Geometry: final body of the model. Coordinates: model frame, mm. A direction names the side the tool comes from. Coordinates: 2 decimals unless noted, no trailing zeros. Loops run counter-clockwise (first coordinate to the right, second up) from the corner with the lowest first, then second, coordinate; pieces in that order, holes last. Notation, with made-up numbers: (10.5, -8) - (31.5, -8) arc R18 cw to (31.5, 8) - close; hole circle Ø11 at (23, 32.5). An arc over 180 degrees is marked (long way). Put each result on its own line as item: value. Start each with the question number.
1) Draft query along Y for faces 5 (the cylindrical face through (0, 3, -22)), 6 (the cylindrical face through (2, 0, -1)), 7 (the flat face through (0, 0, -20)). Return one class per face: +Y half, -Y half, draft (parallel to the pull), parting line (faces both ways), or undercut.
2) Contact query for flat-ended pins moving along their axis: pin 1 Ø3 at (x, y) = (0, 0) entering from +Z; pin 2 Ø3 at (x, z) = (0.5, -19) entering from +Y; pin 3 Ø1.5 at (y, z) = (0.5, -15) entering from +X. Output: stop coordinate, or through.
3) Reachability of faces 1 (the cylindrical face through (0, 2, -28)), 2 (the flat face through (0, 0, -6)), 3 (the cylindrical face through (-3.642, -0.924, 1.117)), 4 (the flat face through (0.1, -2.2, -33)) from +Z, -Z, +X, -X, +Y, -Y: full face, straight path, thin tool, end or side. Return the list, or none.
4) Section B-B on x = 0. Output: boundary loops of the cut face in (y, z).
5) Section A-A on y = 3. Output: boundary loops of the cut face in (x, z), and give its area (3 significant figures).
6) Section C-C on x = -3.5. Output: boundary loops of the cut face in (y, z).
7) Material intervals for line 1 along Z through (x, y) = (0, 3.9); line 2 along Y through (x, z) = (0, -29.75); line 3 along Z through (x, y) = (0.5, -4), sorted ascending. Write a range as from..to.
8) Section D-D on z = -25.5. Output: boundary loops of the cut face in (x, y), and give its area (3 significant figures).
```python
from build123d import *

# Parameters (mm, degrees)
SKETCH1_W                                          = 5.5
SKETCH1_H                                          = 8
SKETCH2_R                                          = 5
BOSS_EXTRUDE1_DEPTH                                = 33
CBORE_FOR_M3_5_HEX_HEAD_MACHINE_SCREW1_D           = 4
CBORE_FOR_M3_5_HEX_HEAD_MACHINE_SCREW1_DEPTH       = 14
CBORE_FOR_M3_5_HEX_HEAD_MACHINE_SCREW1_CBORE_D     = 8.5
CBORE_FOR_M3_5_HEX_HEAD_MACHINE_SCREW1_CBORE_DEPTH = 4
HOLE1_REACH                                        = 38.626
HOLE1_BORE_R                                       = 1
SKETCH6_R                                          = 2
CUT_EXTRUDE1_DEPTH                                 = 10
SKETCH7_R                                          = 2
CUT_EXTRUDE2_DEPTH                                 = 5


with BuildPart() as part:
    # Sketch1 → Revolve1 (revolve)
    with BuildSketch(Plane(origin=(0, 0, 0), x_dir=(1, 0, 0), z_dir=(0, 1, 0))):
        with Locations((2.75, -4)):
            Rectangle(SKETCH1_W, SKETCH1_H)
    revolve(axis=Axis((0, 0, 0), (0, 0, 1)))

    # Sketch2 → Boss-Extrude1 (add)
    with BuildSketch(Plane(origin=(0, 0, 0), x_dir=(-1, 0, 0), z_dir=(0, 0, -1))):
        Circle(SKETCH2_R)
    extrude(amount=BOSS_EXTRUDE1_DEPTH)

    # CBORE for M3.5 Hex Head Machine Screw1
    with Locations(Plane.XY.offset(8)):
        with Locations((0, 0)):
            CounterBoreHole(CBORE_FOR_M3_5_HEX_HEAD_MACHINE_SCREW1_D / 2, CBORE_FOR_M3_5_HEX_HEAD_MACHINE_SCREW1_CBORE_D / 2, CBORE_FOR_M3_5_HEX_HEAD_MACHINE_SCREW1_CBORE_DEPTH, depth=CBORE_FOR_M3_5_HEX_HEAD_MACHINE_SCREW1_DEPTH)

    # Hole1 bore (on position points) → Hole1 (cut, up to next)
    with BuildSketch(Plane(origin=(-5.5, 0, 1.5), x_dir=(0, -1, 0), z_dir=(-1, 0, 0)), mode=Mode.PRIVATE) as hole1_sk1:
        Circle(HOLE1_BORE_R)
    hole1_tool1 = extrude(hole1_sk1.sketch, amount=-HOLE1_REACH, mode=Mode.PRIVATE) & part.part
    add(hole1_tool1.solids().sort_by_distance((-5.5, 0, 1.5))[0], mode=Mode.SUBTRACT)

    # Sketch6 → Cut-Extrude1 (cut)
    with BuildSketch(Plane(origin=(0, 0, -33), x_dir=(-1, 0, 0), z_dir=(0, 0, -1))):
        with Locations(Location((0, 0, 0), (0, 0, 180))):
            Circle(SKETCH6_R)
    extrude(amount=-CUT_EXTRUDE1_DEPTH, mode=Mode.SUBTRACT)

    # Sketch7 → Cut-Extrude2 (cut)
    with BuildSketch(Plane(origin=(0, 5, 0), x_dir=(1, 0, 0), z_dir=(0, 1, 0))):
        with Locations(Location((0, 20, 0), (0, 0, 270))):
            Circle(SKETCH7_R)
    extrude(amount=-CUT_EXTRUDE2_DEPTH, mode=Mode.SUBTRACT)


solid = part.part
```
Answer block:
1. face 5: draft
1. face 6: undercut
1. face 7: +Y half
2. pin 1: stops at z = -6
2. pin 2: stops at y = 5
2. pin 3: stops at x = 5
3. face 1: -Z
3. face 2: +Z
3. face 3: -X
3. face 4: -Z, +X, -X, +Y, -Y
4. outline: (-5.5, 0) - (-5, 0) - (-5, -33) - (-2, -33) - (-2, -23) - (2, -23) - (2, -33) - (5, -33) - (5, -22) - (0, -22) - (0, -18) - (5, -18) - (5, 0) - (5.5, 0) - (5.5, 8) - (4.25, 8) - (4.25, 4) - (2, 4) - (2, -6) - (-2, -6) - (-2, 4) - (-4.25, 4) - (-4.25, 8) - (-5.5, 8) - close
5. outline: (-4.61, 0) - (-4, 0) - (-4, -33) - (4, -33) - (4, 0) - (4.61, 0) - (4.61, 8) - (3.01, 8) - (3.01, 4) - (-3.01, 4) - (-3.01, 8) - (-4.61, 8) - close; hole circle Ø4 at (0, -20)
5. area: 301 mm²
6. outline: (-4.24, 0) - (-3.57, 0) - (-3.57, -33) - (3.57, -33) - (3.57, 0) - (4.24, 0) - (4.24, 8) - (2.41, 8) - (2.41, 4) - (-2.41, 4) - (-2.41, 8) - (-4.24, 8) - close; hole circle Ø2 at (0, 1.5)
7. line 1: z = -33..-22, -18..4
7. line 2: y = -5..-2, 2..5
7. line 3: z = -33..4
8. outline: circle Ø10 at (0, 0); hole circle Ø4 at (0, 0)
8. area: 66.0 mm²
